Geometry check sheet. Reference: drawing and pictorial views, mm from the part's lowest x, y, z. Give positions to 0.01 mm unless a question says otherwise; leave off trailing zeros. Loops run counter-clockwise (first coordinate to the right, second up) from the corner with the lowest first, then second, coordinate; pieces in that order, holes last. Notation, with made-up numbers: (-20, 46.5) -> (20, 46.5) arc R16 ccw to (20, 64.5) -> close; hole circle Ø7 at (61, 33.5). An arc over 180 degrees is marked (long way). One line per item, written item: value. Start each with the question number.
(1) Sectioned sample at C-C, the plane z = 7. Record the cut outline in (x, y).
(2) Sectioned sample at A-A, the plane x = 10. Record the cut outline in (y, z).
(3) Gauge pin test, flat ends, axial feed: pin 1 Ø2.5 at (x, z) = (10, 4.88) entering from +Y; pin 2 Ø0.6 at (y, z) = (0.5, 4.5) entering from +X (1 decimal); pin 3 Ø5 at (x, z) = (5, 8) entering from +Y (1 decimal); pin 4 Ø2 at (x, z) = (2, 7.5) entering from +Y (1 decimal). Record the tip position at first contact, or that the pin passes through.
(4) Scan lines: line 1 along Y through (x, z) = (2, 4.75) (1 decimal); line 2 along X through (y, z) = (17, 8) (1 decimal); line 3 along X through (y, z) = (8.25, 7). Record each from-to range of solid material in increasing order. Write a range as from..to.
(5) Sectioned sample at D-D, the plane x = 12.25. Record the cut outline in (y, z).
(6) Sectioned sample at B-B, the plane z = 3.5. Record the cut outline in (x, y).
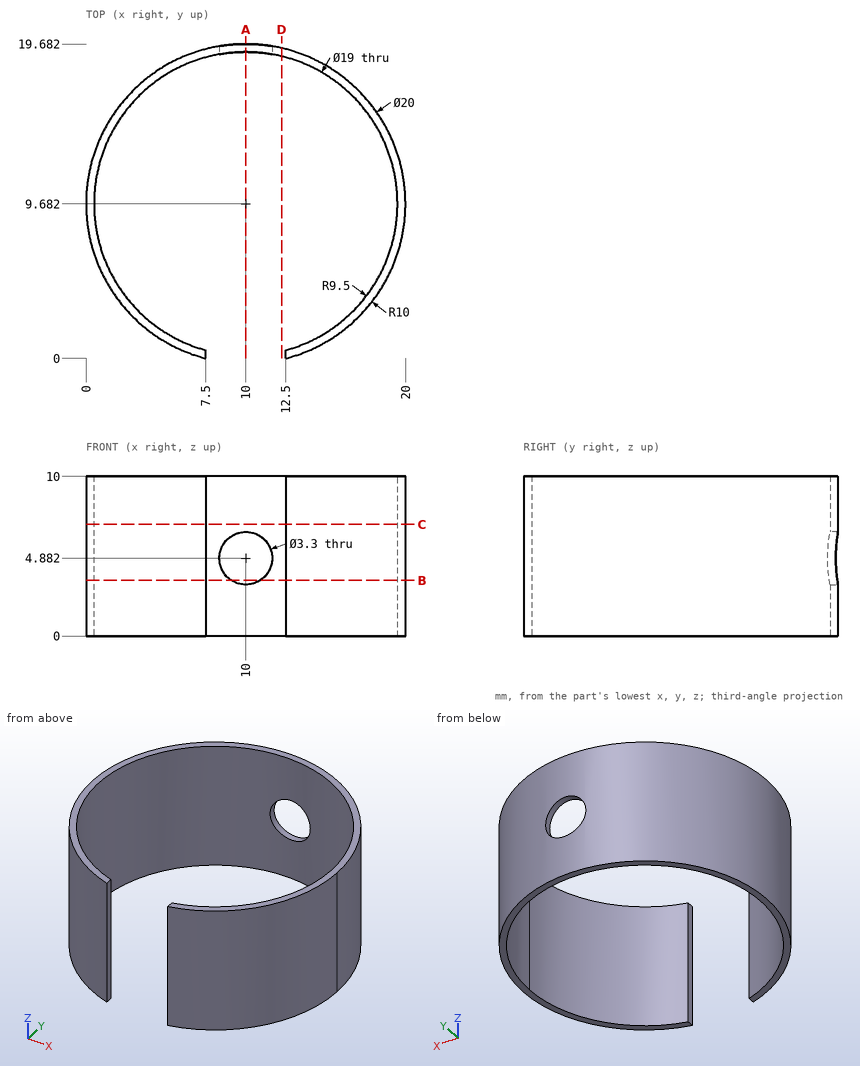
Calculated:
1. outline: (7.5, 0) -> (7.5, 0.52) arc R9.5 cw (long way) to (12.5, 0.52) -> (12.5, 0) arc R10 ccw (long way) to start
2. outline: (19.18, 0) -> (19.68, 0) -> (19.68, 3.23) -> (19.18, 3.23) -> close; (19.18, 6.53) -> (19.68, 6.53) -> (19.68, 10) -> (19.18, 10) -> close
3. pin 1: passes through
3. pin 2: stops at x = 14.6
3. pin 3: stops at y = 19.4
3. pin 4: stops at y = 16.8
4. line 1: y = 3.7..4.6, 14.8..15.7
4. line 2: x = 3.2..3.9, 16.1..16.8
4. line 3: x = 0.1..0.61, 19.39..19.9
5. outline: (18.91, 0) -> (19.43, 0) -> (19.43, 10) -> (18.91, 10) -> close
6. outline: (7.5, 0) -> (7.5, 0.52) arc R9.5 cw to (9.1, 19.14) -> (9.1, 19.64) arc R10 ccw to start; (10.9, 19.14) arc R9.5 cw to (12.5, 0.52) -> (12.5, 0) arc R10 ccw to (10.9, 19.64) -> close
